from build123d import *

# Parameters (mm, degrees)
F0_W      = 38.1
F0_H      = 38.1
F1_DEPTH  = 38.1
F5_DEPTH  = 50.8
F7_DEPTH  = 127
F9_DEPTH  = 50.8
F10_W     = 25.4
F10_H     = 7.62
F11_DEPTH = 50.8


with BuildPart() as f1:
    # F0 (on Front) → F1 (new body)
    with BuildSketch(Plane.XZ):
        with Locations((19.05, 19.05)):
            Rectangle(F0_W, F0_H)
    extrude(amount=F1_DEPTH)

    # F4 (on face) → F5 (cut)
    with BuildSketch(Plane.YZ.offset(38.1)):
        Polygon((-11.4268120378, 38.1), (-31.75, 38.1), (-26.67, 17.145), (-21.59, 28.575), (-16.51, 28.575), (-11.4268120378, 15.875), (-6.3468120378, 38.1), align=None)
        Polygon((-38.1, 0), (-31.75, 0), (-38.1, 38.1), align=None)
        Polygon((-19.05, 15.875), (-25.4, 0), (-12.7, 0), align=None)
        Polygon((0, 38.1), (-6.35, 0), (0, 0), align=None)
    extrude(amount=-F5_DEPTH, mode=Mode.SUBTRACT)

    # F6 (on offset) → F7 (cut)
    with BuildSketch(Plane.XZ.offset(38.1)):
        Polygon((11.43, 22.225), (6.35, 0), (11.43, 0), (26.67, 0), (31.75, 0), (26.4095281363, 22.225), (21.4223176855, 9.558487687), (18.8823176855, 9.558487687), (16.3423176855, 9.558487687), align=None)
        Polygon((18.8823176855, 38.1), (12.7131294711, 38.1), (18.8823176855, 22.258487687), align=None)
        Polygon((25.3863393215, 38.1), (18.8823176855, 38.1), (18.8823176855, 22.258487687), align=None)
        Polygon((31.7556646041, 38.1), (38.1, 0), (38.1, 38.1), align=None)
        Polygon((0, 38.1), (0, 0), (6.3445118444, 38.1), align=None)
    extrude(amount=-F7_DEPTH, mode=Mode.SUBTRACT)

    # F8 (on offset) → F9 (cut)
    with BuildSketch(Plane.XY.offset(38.1)):
        Polygon((12.7, -22.86), (0, -22.86), (0, -30.48), (12.7, -30.48), (25.4, -30.48), (25.4, -22.86), align=None)
    extrude(amount=-F9_DEPTH, mode=Mode.SUBTRACT)

    # F10 (on offset) → F11 (cut)
    with BuildSketch(Plane.XY.offset(38.1)):
        with Locations((25.4, -11.43)):
            Rectangle(F10_W, F10_H)
    extrude(amount=-F11_DEPTH, mode=Mode.SUBTRACT)


solid = f1.part
Work out the finished part from the listing and answer in its coordinate system (mm). A direction names the side the tool comes from. Give positions to 0.01 mm unless a question says otherwise; leave off trailing zeros. Write each loop counter-clockwise with the first axis right and the second up, starting at its lowest first coordinate (ties: lowest second). Pieces come first, ordered by that corner, then holes.
Q1. Straight lines are drawn through the part: L1, parallel to X at y = -4.5, z = 16; L2, parallel to Y at x = 9, z = 24; L3, parallel to Y at x = 33.5, z = 19.5. For each, find the intervals that lie inside material, in ascending order.
Answer:
L1: x = 2.66 to 10.01, 13.84 to 23.96, 27.91 to 35.44
L2: y = -35.75 to -30.48, -22.86 to -14.68, -9.57 to -2.35
L3: y = -35 to -27.24, -25.62 to -15.24, -7.62 to -3.1
Q2. Given pin 1 (5 mm diameter, centred on x = 4.5, y = -21.5, fed in from +Z) (3 decimals); pin 2 (6 mm diameter, centred on x = 18, z = 16, fed in from -Y); pin 3 (1 mm diameter, centred on x = 16, y = -14, fed in from -Z); pin 4 (0.6 mm diameter, centred on x = 19.5, y = -22, fed in from -Z), each flat-ended and moving along its own axis, determine where each tip first touches the part or whether it passes through.
Answer:
pin 1: stops at z = 28.575
pin 2: stops at y = -34.92
pin 3: passes through
pin 4: stops at z = 9.56
Q3. The part is cut by section C-C on y = -7. Give the vertices of the cut face in (x, z) (3 decimals).
Answer:
outline: (0, 0) - (6.35, 0) - (11.43, 22.225) - (16.342, 9.558) - (21.422, 9.558) - (26.41, 22.225) - (31.75, 0) - (38.1, 0) - (32.232, 35.242) - (24.213, 35.242) - (18.882, 22.258) - (13.826, 35.242) - (5.869, 35.242) - close
Q4. For a pull along Y with two mould halves and no side action, classify faces 1 (the face through (19, -20, 13.5)), 2 (the face through (19.32, -34.88, 18.78)), 3 (the face through (19.32, -3.13, 19.32)), 4 (the face through (19, -22, 9.558)) as released by +Y, released by -Y, zero draft, split by the parting line, or undercut.
Answer:
face 1: undercut
face 2: released by -Y
face 3: released by +Y
face 4: zero draft
Q5. The part is cut by section B-B on z = 5. Give the vertices of the cut face in (x, y).
Answer:
outline: (0.83, -32.58) - (7.49, -32.58) - (7.49, -30.48) - (0.83, -30.48) - close; (0.83, -14.7) - (7.49, -14.7) - (7.49, -5.52) - (0.83, -5.52) - close; (30.55, -32.58) - (37.27, -32.58) - (37.27, -23.4) - (30.55, -23.4) - close; (30.55, -7.62) - (37.27, -7.62) - (37.27, -5.52) - (30.55, -5.52) - close
Q6. The part is cut by section A-A on x = 34.5. Give the vertices of the cut face in (y, z) (3 decimals).
Answer:
outline: (-35.353, 21.619) - (-31.75, 0) - (-25.4, 0) - (-19.05, 15.875) - (-15.24, 6.35) - (-15.24, 21.619) - (-24.681, 21.619) - (-26.67, 17.145) - (-27.755, 21.619) - close; (-7.62, 0) - (-6.35, 0) - (-2.747, 21.619) - (-7.62, 21.619) - close
Q7. The part is cut by section D-D on z = 33.5. Give the vertices of the cut face in (x, y).
Answer:
outline: (5.58, -37.33) - (14.5, -37.33) - (14.5, -30.63) - (5.58, -30.63) - close; (5.58, -7.4) - (14.5, -7.4) - (14.5, -0.77) - (5.58, -0.77) - close; (23.5, -37.33) - (32.52, -37.33) - (32.52, -30.63) - (23.5, -30.63) - close; (23.5, -7.4) - (32.52, -7.4) - (32.52, -0.77) - (23.5, -0.77) - close
Q8. A tool of negligible diameter and unlimited length cuts with its end or side. For faces 5 (the face through (13.4, -22.86, 18.3)), 6 (the face through (9, -35, 38.1)), 7 (the face through (11.002, -22.234, 27.126)), 8 (the face through (9.49, -32.45, 13.74)), 9 (the face through (18.97, -18.05, 13.37)), from which of +Z, -Z, +X, -X, +Y, -Y can it reach the whole face along a straight path? Write none if from no direction.
Answer:
face 5: +Z, -Z, -X
face 6: +Z, +X, -X, +Y, -Y
face 7: +Z, +X, -X
face 8: -Z, +Y, -Y
face 9: -Z, +X, -X
